from build123d import *

# Parameters (mm, degrees)
SKETCH2_R           = 2
BOSS_EXTRUDE1_DEPTH = 24
SKETCH3_R           = 1.55
CUT_EXTRUDE1_DEPTH  = 10


with BuildPart() as part:
    # Sketch1 → Revolve1 (revolve)
    with BuildSketch(Plane.XY):
        Polygon((-85, 0), (-85, 55), (-80, 60), (-80, 56), (-70, 56), (-70, 52), (-81, 52), (-81, 0), align=None)
    revolve(axis=Axis((0, -62.463486945, 0), (0, 1, 0)))

    # Sketch2 → Boss-Extrude1 (add)
    with BuildSketch(Plane.XZ):
        with BuildLine():
            ThreePointArc((-43.428412772, 68.37377395), (-35, 60.621778265), (-37.499218807, 71.796995681))
            ThreePointArc((-37.499218807, 71.796995681), (-40.5, 70.148057707), (-43.428412772, 68.37377395))
        make_face()
        with Locations((-38, 65.817930688)):
            Circle(SKETCH2_R, mode=Mode.SUBTRACT)
        with BuildLine():
            ThreePointArc((-43.428412772, -68.37377395), (-40.5, -70.148057707), (-37.499218807, -71.796995681))
            ThreePointArc((-37.499218807, -71.796995681), (-35, -60.621778265), (-43.428412772, -68.37377395))
        make_face()
        with Locations((-38, -65.817930688)):
            Circle(SKETCH2_R, mode=Mode.SUBTRACT)
        with BuildLine():
            ThreePointArc((81, 0), (80.981905874, 1.711993298), (80.927631579, 3.423221731))
            ThreePointArc((80.927631579, 3.423221731), (70, 0), (80.927631579, -3.423221731))
            ThreePointArc((80.927631579, -3.423221731), (80.981905874, -1.711993298), (81, 0))
        make_face()
        with Locations((76, 0)):
            Circle(SKETCH2_R, mode=Mode.SUBTRACT)
    extrude(amount=-BOSS_EXTRUDE1_DEPTH)

    # Sketch3 → Cut-Extrude1 (cut)
    with BuildSketch(Plane(origin=(0, 56, 0), x_dir=(1, 0, 0), z_dir=(0, 1, 0))):
        with Locations((-64.951905284, -37.5)):
            Circle(SKETCH3_R)
        with Locations((64.951905284, 37.5)):
            Circle(SKETCH3_R)
    extrude(amount=-CUT_EXTRUDE1_DEPTH, mode=Mode.SUBTRACT)


solid = part.part
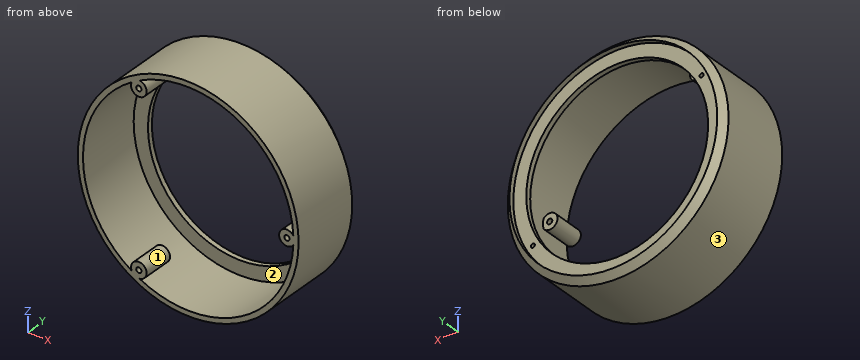
Design review of the part built by this model. Coordinates are the model's own, in mm. Face numbers are marked on the shaded views. Coordinates: 2 decimals unless noted, no trailing zeros. Order: outer loops, then holes, each group sorted by start corner. A loop starts at its lowest first (then second) coordinate and runs counter-clockwise, first axis right, second up. Notation, with made-up numbers: (-24.5, 50.25) -> (10.5, 50.25) arc R15 cw to (10.5, 70.25) -> close; hole circle Ø10 at (34.25, 36.25). An arc over 180 degrees is marked (long way). Use one line per item in the form item = value. Start each with the question number.
(1) The part is to be moulded in two halves that separate along X. For the marked faces 1, 2 and 3, say which applies: +X half, -X half, draft (parallel to the pull), parting line (faces both ways), or undercut.
(2) For probe 1 along X at (y, z) = (5, -62); probe 2 along Z at (x, y) = (0, 53); probe 3 along Y at (x, z) = (-72, 27.5), list the stretches that pass through material, from the lowest coordinate up.
(3) Add section B-B on y = 11. State the section outline as (x, z) points, plus the area to 3 significant figures.
(4) Add section A-A on x = 0. State the section outline as (y, z) points, plus the area to 3 significant figures.
(5) Add section C-C on y = 49.5. State the section outline as (x, z) points, plus the area to 3 significant figures.
(6) Insertion check: pin 1 (3 mm diameter, centred on x = 28.5, y = 45, fed in from +Z); pin 2 (6 mm diameter, centred on x = 34.5, y = 44, fed in from +Z); pin 3 (4 mm diameter, centred on y = 46.5, z = 58.5, fed in from +X). Each pin has a flat end and moves straight along its axis. Give the tip position at first contact, or say it passes through.
Answer block:
q1.face_1 = undercut
q1.face_2 = undercut
q1.face_3 = parting line
q2.probe_1 = -58.15 to -52.12, -42.63 to -33.37, 52.12 to 58.15
q2.probe_2 = -85 to -70, 70 to 85
q2.probe_3 = 52 to 56
q3.outline = circle Ø170 at (0, 0); hole (-43.43, -68.37) arc R6 cw (long way) to (-37.5, -71.8) arc R81 ccw to (80.93, -3.42) arc R6 cw (long way) to (80.93, 3.42) arc R81 ccw to (-37.5, 71.8) arc R6 cw (long way) to (-43.43, 68.37) arc R81 ccw to start; hole circle Ø4 at (-38, -65.82); hole circle Ø4 at (-38, 65.82); hole circle Ø4 at (76, 0)
q3.area = 2,370 mm²
q4.outline = (0, -85) -> (55, -85) -> (60, -80) -> (56, -80) -> (56, -70) -> (52, -70) -> (52, -81) -> (0, -81) -> close; (0, 81) -> (52, 81) -> (52, 70) -> (56, 70) -> (56, 80) -> (60, 80) -> (55, 85) -> (0, 85) -> close
q4.area = 551 mm²
q5.outline = circle Ø170 at (0, 0); hole circle Ø162 at (0, 0)
q5.area = 2,090 mm²
q6.pin_1 = 80.6
q6.pin_2 = 78.95
q6.pin_3 = 63.5
